Build history of the part. All positions in model axes, mm. Give positions to 0.01 mm unless a question says otherwise; leave off trailing zeros. Order: outer loops, then holes, each group sorted by start corner. A loop starts at its lowest first (then second) coordinate and runs counter-clockwise, first axis right, second up. Notation, with made-up numbers: (89.25, 10) - (115.25, 10) arc R18 ccw to (115.25, 23) - close; hole circle Ø2 at (30, -7.75). An arc over 180 degrees is marked (long way). One line per item, written item: value.
```python
from build123d import *

# Parameters (mm, degrees)
SKETCH_1_R      = 2.025
EXTRUDE_1_DEPTH = 4


with BuildPart() as part:
    # 草图1 → 凸台-拉伸1 (new body)
    with BuildSketch(Plane.XY):
        with BuildLine():
            Line((-98, -32.5), (98, -32.5))
            ThreePointArc((98, -32.5), (102.057826292, -29.945262394), (101.508238617, -25.181798126))
            ThreePointArc((101.508238617, -25.181798126), (93.492529314, -10.937801768), (90.498696296, 5.130178558))
            ThreePointArc((90.498696296, 5.130178558), (88.549936229, 9.641990986), (84, 11.5))
            Line((84, 11.5), (69, 11.5))
            ThreePointArc((69, 11.5), (63.988927391, 9.13994581), (62.616747985, 3.773585019))
            ThreePointArc((62.616747985, 3.773585019), (58.39465774, -12.73829462), (42.975972641, -20))
            Line((42.975972641, -20), (-42.975972641, -20))
            ThreePointArc((-42.975972641, -20), (-58.394657646, -12.738294733), (-62.61674804, 3.773584731))
            ThreePointArc((-62.61674804, 3.773584731), (-63.988927298, 9.139945697), (-69, 11.5))
            Line((-69, 11.5), (-84, 11.5))
            ThreePointArc((-84, 11.5), (-88.549936232, 9.641990982), (-90.498696296, 5.130178548))
            ThreePointArc((-90.498696296, 5.130178548), (-93.492529331, -10.937801814), (-101.508238673, -25.181798195))
            ThreePointArc((-101.508238673, -25.181798195), (-102.057826273, -29.945262434), (-98, -32.5))
        make_face()
        with Locations((-84, -28)):
            Circle(SKETCH_1_R, mode=Mode.SUBTRACT)
        with Locations((84, -5)):
            Circle(SKETCH_1_R, mode=Mode.SUBTRACT)
        with Locations((69, -5)):
            Circle(SKETCH_1_R, mode=Mode.SUBTRACT)
        with Locations((-70, -28)):
            Circle(SKETCH_1_R, mode=Mode.SUBTRACT)
        with Locations((-56, -28)):
            Circle(SKETCH_1_R, mode=Mode.SUBTRACT)
        with Locations((-42, -28)):
            Circle(SKETCH_1_R, mode=Mode.SUBTRACT)
        with Locations((-28, -28)):
            Circle(SKETCH_1_R, mode=Mode.SUBTRACT)
        with Locations((-14, -28)):
            Circle(SKETCH_1_R, mode=Mode.SUBTRACT)
        with Locations((0, -28)):
            Circle(SKETCH_1_R, mode=Mode.SUBTRACT)
        with Locations((14, -28)):
            Circle(SKETCH_1_R, mode=Mode.SUBTRACT)
        with Locations((28, -28)):
            Circle(SKETCH_1_R, mode=Mode.SUBTRACT)
        with Locations((42, -28)):
            Circle(SKETCH_1_R, mode=Mode.SUBTRACT)
        with Locations((56, -28)):
            Circle(SKETCH_1_R, mode=Mode.SUBTRACT)
        with Locations((70, -28)):
            Circle(SKETCH_1_R, mode=Mode.SUBTRACT)
        with Locations((-84, -5)):
            Circle(SKETCH_1_R, mode=Mode.SUBTRACT)
        with Locations((-69, -5)):
            Circle(SKETCH_1_R, mode=Mode.SUBTRACT)
        with Locations((84, -28)):
            Circle(SKETCH_1_R, mode=Mode.SUBTRACT)
        with Locations((-98, -28)):
            Circle(SKETCH_1_R, mode=Mode.SUBTRACT)
        with Locations((-84, 5)):
            Circle(SKETCH_1_R, mode=Mode.SUBTRACT)
        with Locations((98, -28)):
            Circle(SKETCH_1_R, mode=Mode.SUBTRACT)
        with Locations((-69, 5)):
            Circle(SKETCH_1_R, mode=Mode.SUBTRACT)
        with Locations((84, 5)):
            Circle(SKETCH_1_R, mode=Mode.SUBTRACT)
        with Locations((69, 5)):
            Circle(SKETCH_1_R, mode=Mode.SUBTRACT)
    extrude(amount=EXTRUDE_1_DEPTH)


solid = part.part
```
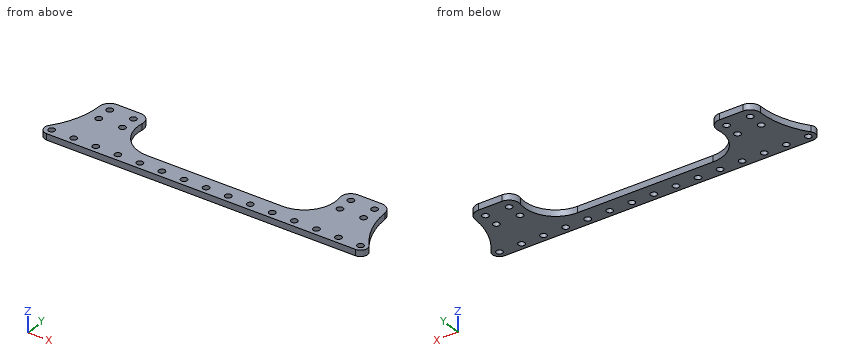
(1) Slice it at C-C, the plane y = -5. Give the cut face in (x, z) (3 decimals).
Completed:
outline: (-91.744, 0) - (-86.025, 0) - (-86.025, 4) - (-91.744, 4) - close; (-81.975, 0) - (-71.025, 0) - (-71.025, 4) - (-81.975, 4) - close; (-66.975, 0) - (-62.341, 0) - (-62.341, 4) - (-66.975, 4) - close; (62.341, 0) - (66.975, 0) - (66.975, 4) - (62.341, 4) - close; (71.025, 0) - (81.975, 0) - (81.975, 4) - (71.025, 4) - close; (86.025, 0) - (91.744, 0) - (91.744, 4) - (86.025, 4) - close
(2) Slice it at D-D, the plane x = 56. Give the cut face in (y, z) (3 decimals).
Completed:
outline: (-32.5, 0) - (-30.025, 0) - (-30.025, 4) - (-32.5, 4) - close; (-25.975, 0) - (-15.178, 0) - (-15.178, 4) - (-25.975, 4) - close
(3) Pin check, flat tips, straight feed: P1, Ø6.5, axis at x = 42, y = -28, coming from the -Z side; P2, Ø2, axis at x = 11, z = 3, coming from the +Y side. Stop position of each tip, or through.
Completed:
P1: z = 0
P2: y = -20
(4) Slice it at A-A, the plane x = 0. Give the cut face in (y, z) (3 decimals).
Completed:
outline: (-32.5, 0) - (-30.025, 0) - (-30.025, 4) - (-32.5, 4) - close; (-25.975, 0) - (-20, 0) - (-20, 4) - (-25.975, 4) - close
(5) Slice it at B-B, the plane y = -28. Count the separate pieces of the cut face and the enclosed holes in it, and give its area (3 significant figures).
Completed:
separate pieces: 16
enclosed holes: 0
area: 577 mm²
(6) Drill centre lines: line 1 (Y direction, x = -84, z = 2.75) (3 decimals); line 2 (Y direction, x = -42, z = 2.7) (3 decimals); line 3 (X direction, y = 6, z = 1.55). Where is each one in solid material? Low to high.
Completed:
line 1: -32.5 to -30.025, -25.975 to -7.025, -2.975 to 2.975, 7.025 to 11.5
line 2: -32.5 to -30.025, -25.975 to -20
line 3: -90.42 to -85.76, -82.24 to -70.76, -67.24 to -62.58, 62.58 to 67.24, 70.76 to 82.24, 85.76 to 90.42
